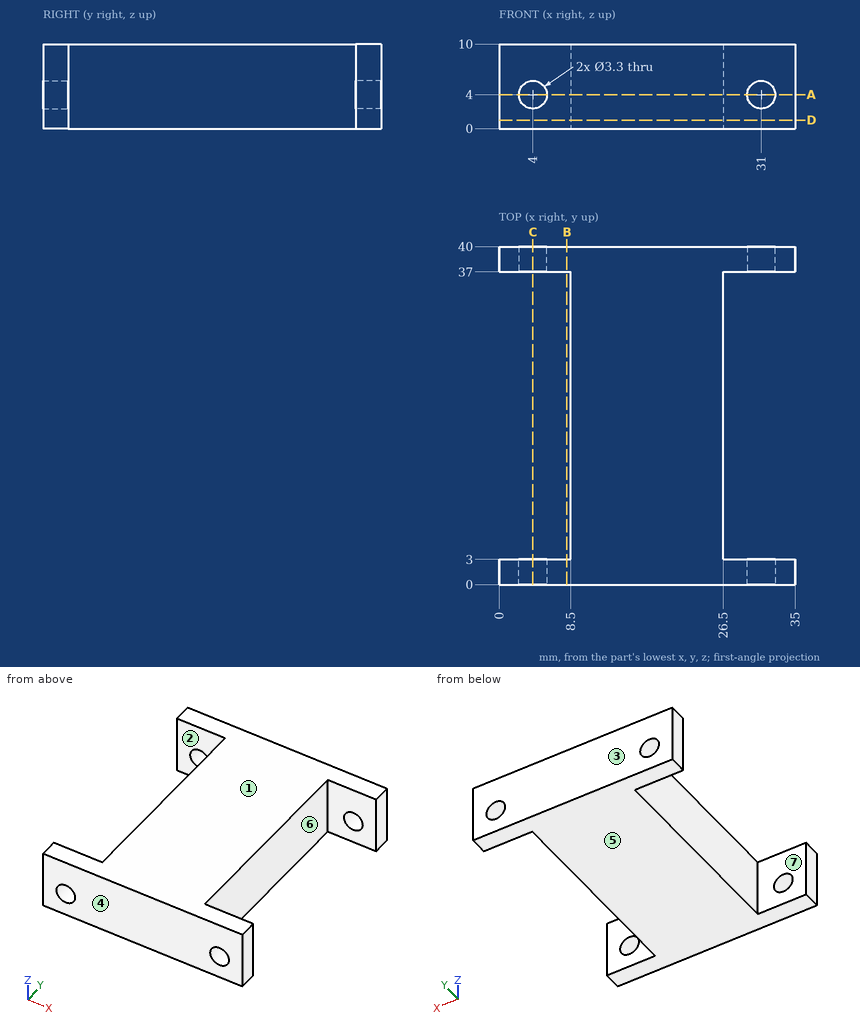
Check sheet for the drawn part. Datum: minimum x, y, z corner. Units: mm. A direction names the side the tool comes from. Round coordinates to 2 decimals unless told otherwise and drop trailing zeros. Write each loop counter-clockwise with the first axis right and the second up, starting at its lowest first coordinate (ties: lowest second). Pieces come first, ordered by that corner, then holes. Notation, with made-up numbers: (12.25, 3) - (62.25, 3) arc R9 ccw to (62.25, 9) - close; hole circle Ø11 at (66, -10). An arc over 180 degrees is marked (long way). Return JSON: item names as keys, results as strings.
Q1. Scan lines: L1, parallel to X at y = 1.4, z = 4; L2, parallel to Z at x = 4, y = 2; L3, parallel to Y at x = 2, z = 8.25. Record each from-to range of solid material in increasing order. Write a range as from..to.
Returned:
{"L1": "x = 0..2.35, 5.65..29.35, 32.65..35", "L2": "z = 0..2.35, 5.65..10", "L3": "y = 0..3, 37..40"}
Q2. Depth check by flat-ended pin: P1, Ø4.5, axis at x = 31, z = 4, coming from the +Y side; P2, Ø3, axis at x = 31, z = 4, coming from the -Y side; P3, Ø3, axis at y = 23.5, z = 6, coming from the -X side; P4, Ø5, axis at y = 22.5, z = 3, coming from the +X side. Enter the tip coordinate at first touch or a pass-through.
Returned:
{"P1": "stops at y = 40", "P2": "passes through", "P3": "stops at x = 8.5", "P4": "stops at x = 26.5"}
Q3. Cross-section at D-D (z = 1). Record the boundary of the cut face in (x, y).
Returned:
{"outline": "(0, 0) - (35, 0) - (35, 3) - (26.5, 3) - (26.5, 37) - (35, 37) - (35, 40) - (0, 40) - (0, 37) - (8.5, 37) - (8.5, 3) - (0, 3) - close"}
Q4. Access from +Z, -Z, +X, -X, +Y, -Y to the whole of each face (thin tool, end or side, straight path). Record for the marked faces 5, 6 and 7.
Returned:
{"face 5": "-Z, +X, -X, +Y, -Y", "face 6": "+Z, -Z, +X", "face 7": "+Z, -Z, -X"}
Q5. Cross-section at A-A (z = 4). Record the boundary of the cut face in (x, y).
Returned:
{"outline": "(0, 0) - (2.35, 0) - (2.35, 3) - (0, 3) - close; (0, 37) - (2.35, 37) - (2.35, 40) - (0, 40) - close; (5.65, 0) - (29.35, 0) - (29.35, 3) - (26.5, 3) - (26.5, 37) - (29.35, 37) - (29.35, 40) - (5.65, 40) - (5.65, 37) - (8.5, 37) - (8.5, 3) - (5.65, 3) - close; (32.65, 0) - (35, 0) - (35, 3) - (32.65, 3) - close; (32.65, 37) - (35, 37) - (35, 40) - (32.65, 40) - close"}
Q6. Cross-section at C-C (x = 4). Record the boundary of the cut face in (y, z), then the cut area to 3 significant figures.
Returned:
{"outline": "(0, 0) - (3, 0) - (3, 2.35) - (0, 2.35) - close; (0, 5.65) - (3, 5.65) - (3, 10) - (0, 10) - close; (37, 0) - (40, 0) - (40, 2.35) - (37, 2.35) - close; (37, 5.65) - (40, 5.65) - (40, 10) - (37, 10) - close", "area": "40.2 mm²"}
Q7. Cross-section at B-B (x = 8). Record the boundary of the cut face in (y, z).
Returned:
{"outline": "(0, 0) - (3, 0) - (3, 10) - (0, 10) - close; (37, 0) - (40, 0) - (40, 10) - (37, 10) - close"}
Q8. Draft check along Y on the marked faces 1, 2, 3 and 4. Enter one of: released by +Y, released by -Y, zero draft, split by the parting line, or undercut.
Returned:
{"face 1": "zero draft", "face 2": "undercut", "face 3": "released by +Y", "face 4": "released by -Y"}
